Model file for the job. Use its own axes, mm. A direction names the side the tool comes from. Round coordinates to 2 decimals unless told otherwise and drop trailing zeros. Write each loop counter-clockwise with the first axis right and the second up, starting at its lowest first coordinate (ties: lowest second). Pieces come first, ordered by that corner, then holes. Notation, with made-up numbers: (5, 77) - (40, 77) arc R30 ccw to (40, 115) - close; hole circle Ø1 at (57, 33). An arc over 180 degrees is marked (long way). Answer as a JSON object with one key per item and string values. Group by question number.
from build123d import *

# Parameters (mm, degrees)
SKETCH43_W           = 140
SKETCH43_H           = 99.999981374
BOSS_EXTRUDE10_DEPTH = 3.175
SKETCH45_W           = 3.175
SKETCH45_H           = 20
SKETCH45_W_2         = 20
SKETCH45_H_2         = 3.175
CUT_EXTRUDE22_DEPTH  = 3.175


with BuildPart() as part:
    # Sketch43 → Boss-Extrude10 (new body)
    with BuildSketch(Plane(origin=(0, 0, 0), x_dir=(0, 0, -1), z_dir=(1, 0, 0))):
        with Locations((-668.101928689, 4.4643e-05)):
            Rectangle(SKETCH43_W, SKETCH43_H)
    extrude(amount=BOSS_EXTRUDE10_DEPTH)

    # Sketch45 → Cut-Extrude22 (cut)
    with BuildSketch(Plane(origin=(3.175, 0, 0), x_dir=(0, 0, -1), z_dir=(1, 0, 0))):
        with Locations((-599.689428689, 20.000053956)):
            Rectangle(SKETCH45_W, SKETCH45_H)
        with Locations((-736.514428689, 20.000053956)):
            Rectangle(SKETCH45_W, SKETCH45_H)
        with Locations((-736.514428689, -19.999946044)):
            Rectangle(SKETCH45_W, SKETCH45_H)
        with Locations((-599.689428689, -19.999946044)):
            Rectangle(SKETCH45_W, SKETCH45_H)
        with Locations((-668.101928689, -48.412446044)):
            Rectangle(SKETCH45_W_2, SKETCH45_H_2)
        with Locations((-708.101928689, -48.412446044)):
            Rectangle(SKETCH45_W_2, SKETCH45_H_2)
        with Locations((-628.101928689, -48.412446044)):
            Rectangle(SKETCH45_W_2, SKETCH45_H_2)
        with Locations((-668.101928689, 48.41253533)):
            Rectangle(SKETCH45_W_2, SKETCH45_H_2)
        with Locations((-708.101928689, 48.41253533)):
            Rectangle(SKETCH45_W_2, SKETCH45_H_2)
        with Locations((-628.101928689, 48.41253533)):
            Rectangle(SKETCH45_W_2, SKETCH45_H_2)
    extrude(amount=-CUT_EXTRUDE22_DEPTH, mode=Mode.SUBTRACT)


solid = part.part
(1) 3-axis set-ups, long thin cutter, end or side, ignore diameter. For faces 5 (the flat face through (2, 48, 638.102)), 6 (the flat face through (2, 50, 688)), 7 (the flat face through (2, -46.825, 708)), 8 (the flat face through (2, -50, 688)), 9 (the flat face through (2, 20, 734.927)): which of +Z, -Z, +X, -X, +Y, -Y reach the whole face in a straight line?
(2) Slice it at A-A (y = -21.5). Write the cut outline in (x, z) (3 decimals), then the cut area to 3 significant figures.
(3) Pull direction Y, two halves, no side cores. Call faces 1 (the flat face through (2, -30, 600)), 2 (the flat face through (2, -50, 608)), 3 (the flat face through (2, -40, 738.102)), 4 (the flat face through (2, 46.825, 708)): pulls with the +Y half, pulls with the -Y half, needs draft (parallel to the pull), parting line crosses it, or undercut.
(4) Flat gauge pins, fed straight in: pin 1 (1.6 mm diameter, centred on x = 2, y = 24, fed in from +Z); pin 2 (1 mm diameter, centred on x = 1, z = 630.5, fed in from +Y); pin 3 (1.6 mm diameter, centred on x = 1.5, z = 633, fed in from -Y); pin 4 (1 mm diameter, centred on y = 5.5, z = 674.5, fed in from -X). Where does each tip first touch, or does it go through?
(5) Drill centre lines: line 1 (Z direction, x = 2.05, y = 21); line 2 (Y direction, x = 1.8, z = 718). Where is each one in solid material? Low to high. Write a range as from..to.
(6) Slice it at B-B (z = 630). Write the cut outline in (x, y) (3 decimals).
Answer:
{
 "1": {"face 5": "+X, -X, +Y", "face 6": "+Z, -Z, +X, -X, +Y", "face 7": "+X, -X, -Y", "face 8": "+Z, -Z, +X, -X, -Y", "face 9": "+Z, +X, -X"},
 "2": {"outline": "(0, 601.277) - (3.175, 601.277) - (3.175, 734.927) - (0, 734.927) - close", "area": "424 mm²"},
 "3": {"face 1": "undercut", "face 2": "pulls with the -Y half", "face 3": "needs draft", "face 4": "pulls with the +Y half"},
 "4": {"pin 1": "z = 734.93", "pin 2": "y = 46.83", "pin 3": "y = -46.82", "pin 4": "x = 0"},
 "5": {"line 1": "601.28..734.93", "line 2": "-46.82..46.83"},
 "6": {"outline": "(0, -46.825) - (3.175, -46.825) - (3.175, 46.825) - (0, 46.825) - close"}
}
